Source: CAD feature listing. Evaluate the final solid. Frame: model axes, mm. Face numbers are marked on the shaded views. A direction names the side the tool comes from. Give positions to 0.01 mm unless a question says otherwise; leave off trailing zeros. Loops run counter-clockwise (first coordinate to the right, second up) from the corner with the lowest first, then second, coordinate; pieces in that order, holes last. Notation, with made-up numbers: (19.25, 77.5) - (71.25, 77.5) arc R30 ccw to (71.25, 99.5) - close; hole circle Ø11 at (88, 4). An arc over 180 degrees is marked (long way). Write each question's results on one line, items separated by ' | '. Start each with the question number.
(1) Cut plane D-D on z = 53.5. Return the cut outline in (x, y).
(2) Contact query for flat-ended pins moving along their axis: pin 1 (5 mm diameter, centred on y = 6.5, z = 60.5, fed in from -X); pin 2 (2 mm diameter, centred on y = 4.5, z = -10.5, fed in from -X); pin 3 (3 mm diameter, centred on x = 1.5, y = 8, fed in from +Z). Output: stop coordinate, or through.
(3) Pull-direction query (Z, two-part tool) for the marked faces 1 and 2; classes: pulls with the +Z half, pulls with the -Z half, needs draft (parallel to the pull), parting line crosses it, or undercut.
(4) Cut plane A-A on z = -3. Return the cut outline in (x, y), then the cut area to 3 significant figures.
(5) Reachability of the marked faces 3 and 4 from +Z, -Z, +X, -X, +Y, -Y: full face, straight path, thin tool, end or side. Return the list, or none.
(6) Cut plane C-C on y = 4.25. Return the cut outline in (x, z).
(7) Cut plane B-B on x = 3.75. Return the cut outline in (y, z).
(8) Material intervals for line 1 along Z through (x, y) = (4.5, 2.25); line 2 along X through (y, z) = (1.75, -1); line 3 along X through (y, z) = (3.25, 11), sorted ascending. Write a range as [from, to].
from build123d import *

# Parameters (mm, degrees)
BOSS_EXTRUDE1_DEPTH = 11.6586
SKETCH2_5_W         = 3.1369
SKETCH2_5_H         = 0.491550165
CUT_EXTRUDE2_DEPTH  = 79.458628588
CUT_EXTRUDE4_START  = 77.0734
SKETCH3_W           = 1.524
SKETCH3_H           = 5.8293
CUT_EXTRUDE4_DEPTH  = 25.4


with BuildPart() as part:
    # Sketch2 → Boss-Extrude1 (new body)
    with BuildSketch(Plane(origin=(0, 0, 0), x_dir=(1, 0, 0), z_dir=(0, 1, 0))):
        Polygon((0, 5.08), (0, -1.556064247), (5.869646797, -1.556064247), (5.869646797, -77.07340022), (8.917646797, -77.07340022), (8.917646797, 28.173908926), (2.732746797, 28.173908926), (2.732746797, 26.3144), (5.869646797, 26.3144), (5.869646797, 12.6492), (2.732746797, 12.6492), (2.732746797, 0), (1.132546797, 0), (1.132546797, 5.08), align=None)
    extrude(amount=BOSS_EXTRUDE1_DEPTH)

    # Sketch2<5> → Cut-Extrude2 (cut, through all)
    with BuildSketch(Plane(origin=(0, 0, 0), x_dir=(1, 0, 0), z_dir=(0, 1, 0))):
        with Locations((4.301196797, 8.275924918)):
            Rectangle(SKETCH2_5_W, SKETCH2_5_H)
    extrude(amount=CUT_EXTRUDE2_DEPTH, mode=Mode.SUBTRACT)

    # Sketch3 → Cut-Extrude4 (cut)
    with BuildSketch(Plane.XY.offset(CUT_EXTRUDE4_START)):
        with Locations((6.631646797, 5.8293)):
            Rectangle(SKETCH3_W, SKETCH3_H)
    extrude(amount=-CUT_EXTRUDE4_DEPTH, mode=Mode.SUBTRACT)


solid = part.part
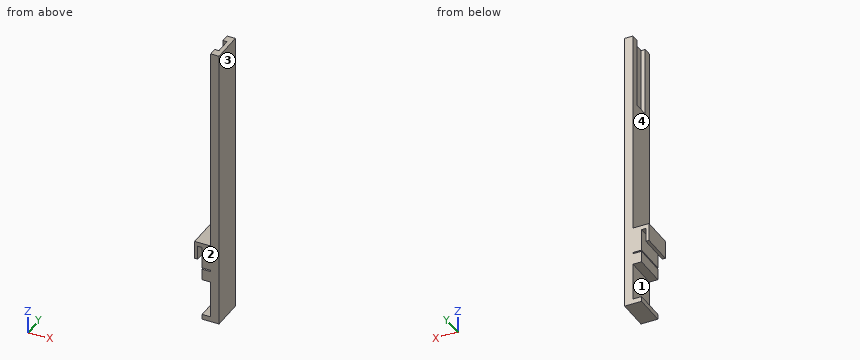
Ans:
1) outline: (5.87, 0) - (8.92, 0) - (8.92, 11.66) - (5.87, 11.66) - (5.87, 8.74) - (7.39, 8.74) - (7.39, 2.91) - (5.87, 2.91) - close
2) pin 1: x = 5.87 | pin 2: x = 2.73 | pin 3: z = 1.56
3) face 1: undercut | face 2: needs draft
4) outline: (0, 0) - (1.13, 0) - (1.13, 11.66) - (0, 11.66) - close; (2.73, 0) - (8.92, 0) - (8.92, 11.66) - (2.73, 11.66) - close | area: 85.3 mm^2
5) face 3: +Z, -Z, +X, +Y, -Y | face 4: +Z, -X, +Y, -Y
6) outline: (0, -5.08) - (1.13, -5.08) - (1.13, 0) - (2.73, 0) - (2.73, -8.03) - (5.87, -8.03) - (5.87, -8.52) - (2.73, -8.52) - (2.73, -12.65) - (5.87, -12.65) - (5.87, -26.31) - (2.73, -26.31) - (2.73, -28.17) - (8.92, -28.17) - (8.92, 77.07) - (7.39, 77.07) - (7.39, 51.67) - (5.87, 51.67) - (5.87, 1.56) - (0, 1.56) - close
7) outline: (0, -28.17) - (11.66, -28.17) - (11.66, -26.31) - (0, -26.31) - close; (0, -12.65) - (11.66, -12.65) - (11.66, -8.52) - (0, -8.52) - close; (0, -8.03) - (11.66, -8.03) - (11.66, 1.56) - (0, 1.56) - close
8) line 1: [-28.17, -26.31], [-12.65, -8.52], [-8.03, 1.56] | line 2: [0, 1.13], [2.73, 8.92] | line 3: [5.87, 8.92]
